Autodesk Inventor part; units mm, degrees
ref_plane "YZ Plane" through (0, 0, 0) normal (1, 0, 0) x (0, 1, 0)
ref_plane "XZ Plane" through (0, 0, 0) normal (0, 1, 0) x (-1, 0, 0)
ref_plane "XY Plane" through (0, 0, 0) normal (0, 0, 1) x (1, 0, 0)
sketch "Sketch1" plane through (0, 0, 0) normal (0, 0, 1) x (1, 0, 0)
  line L0 (6, 1.5) -> (6, -1.5)
  line L1 (8, 0.5) -> (11.5, 0.5)
  line L2 (12.5, 1.5) -> (12.5, 2.3)
  line L3 (12.5, 1.5) -> (11.5, 1.5) construction
  line L4 (11.5, 1.5) -> (11.5, 0.5) construction
  arc A0 (11.5, 0.5) -> (12.5, 1.5) centre (11.5, 1.5) ccw
  line L5 (6, 1.5) -> (9.5, 1.5)
  line L6 (12.5, 2.3) -> (9.5, 2.3)
  line L7 (9.5, 2.3) -> (9.5, 1.5)
  line L8 (8, -0.5) -> (8, 0.5)
  line L9 (6, -2.5) -> (8, -2.5)
  line L10 (8, -2.5) -> (8, -0.5)
  line L11 (0, 0) -> (0, 11.9081) construction
  line L12 (6, -2.5) -> (6, -1.5)
  dimension "d0" = 3
  dimension "d1" = 1.5
  dimension "d2" = 0.8
  dimension "d3" = 1
  dimension "d4" = 1
  dimension "d5" = 3
  dimension "d6" = 6
  dimension "d7" = 0.8
  dimension "d8" = 3.5
  dimension "d11" = 1
revolve "Revolution1" add sketch "Sketch1" angle 360 about axis through (0, 0, 0) along (0, 1, 0)
equation "\"d1\" = 0.5 * d0"
equation "\"d4\" = d3"
properties part number "tarcza sprzęgła 2"
The listing builds one solid part. Answer for the finished solid, in the listing's coordinates (mm). A direction names the side the tool comes from. Coordinates: 2 decimals unless noted, no trailing zeros. Write each loop counter-clockwise with the first axis right and the second up, starting at its lowest first coordinate (ties: lowest second). Pieces come first, ordered by that corner, then holes. Notation, with made-up numbers: (-32.5, 25) - (21.5, 25) arc R26 ccw to (21.5, 39) - close; hole circle Ø6 at (82.5, 56). An arc over 180 degrees is marked (long way). Return JSON: item names as keys, results as strings. Group by question number.
Q1. The part is cut by section D-D on y = 1. Write down the section's boundary in (x, z), and give its area (3 significant figures).
Q2. Flat-ended cylindrical pins translate along their axes: pin 1 Ø12 at (x, z) = (-2.5, 1.5) entering from +Y; pin 2 Ø1 at (y, z) = (0.5, -9.5) entering from +X; pin 3 Ø1 at (x, y) = (2.5, -2) entering from +Z; pin 4 Ø15 at (x, z) = (-4.5, 0) entering from +Y. Find the tip coordinate at first contact, or state that the pin passes through.
Q3. The part is cut by section A-A on x = 0. Write down the section's boundary in (y, z), and give its area (3 significant figures).
Q4. The part is cut by section C-C on y = -0.85. Write down the section's boundary in (x, z), and give its area (3 significant figures).
Q5. For a pull along X with two mould halves and no side action, classify faces 4 (the cylindrical face through (-6, 0, 0)), 5 (the flat face through (-8, 0.5, 2)), 6 (the cylindrical face through (11.923, 1.906, -3.755)), 7 (the cylindrical face through (4.38, 1.89, -8.43)) as +X half, -X half, draft (parallel to the pull), parting line (faces both ways), or undercut.
Q6. The part is cut by section B-B on z = 0. Write down the section's boundary in (x, y), and give its area (3 significant figures).
Q7. Which of the six approach directions +Z, -Z, +X, -X, +Y, -Y give full straight-line access (tool end or side, diameter ignored) to faces 1 (the flat face through (-0.1, 1.5, 6.2)), 2 (the flat face through (2.7, 2.3, -9.3)), 3 (the cylindrical face through (-1.73, -0.98, 7.81))?
Q8. Find the intervals of material crossed by line 1 along X through (y, z) = (1.9, 0); line 2 along Z through (x, y) = (0, -0.9), in increasing order. Write a range as [from, to].
Evaluation:
{
 "1": {"outline": "circle Ø24.73 at (0, 0); hole circle Ø12 at (0, 0)", "area": "367 mm2"},
 "2": {"pin 1": "stops at y = 1.5", "pin 2": "stops at x = 8.17", "pin 3": "stops at z = 7.75", "pin 4": "stops at y = 2.3"},
 "3": {"outline": "(-2.5, -8) - (0.5, -8) - (0.5, -11.5) arc R1 ccw to (1.5, -12.5) - (2.3, -12.5) - (2.3, -9.5) - (1.5, -9.5) - (1.5, -6) - (-2.5, -6) - close; (-2.5, 6) - (1.5, 6) - (1.5, 9.5) - (2.3, 9.5) - (2.3, 12.5) - (1.5, 12.5) arc R1 ccw to (0.5, 11.5) - (0.5, 8) - (-2.5, 8) - close", "area": "29.4 mm2"},
 "4": {"outline": "circle Ø16 at (0, 0); hole circle Ø12 at (0, 0)", "area": "88.0 mm2"},
 "5": {"face 4": "undercut", "face 5": "draft", "face 6": "parting line", "face 7": "undercut"},
 "6": {"outline": "(-12.5, 1.5) arc R1 ccw to (-11.5, 0.5) - (-8, 0.5) - (-8, -2.5) - (-6, -2.5) - (-6, 1.5) - (-9.5, 1.5) - (-9.5, 2.3) - (-12.5, 2.3) - close; (6, -2.5) - (8, -2.5) - (8, 0.5) - (11.5, 0.5) arc R1 ccw to (12.5, 1.5) - (12.5, 2.3) - (9.5, 2.3) - (9.5, 1.5) - (6, 1.5) - close", "area": "29.4 mm2"},
 "7": {"face 1": "+Y", "face 2": "+Z, -Z, +X, -X, +Y", "face 3": "-Y"},
 "8": {"line 1": "x = [-12.5, -9.5], [9.5, 12.5]", "line 2": "z = [-8, -6], [6, 8]"}
}
